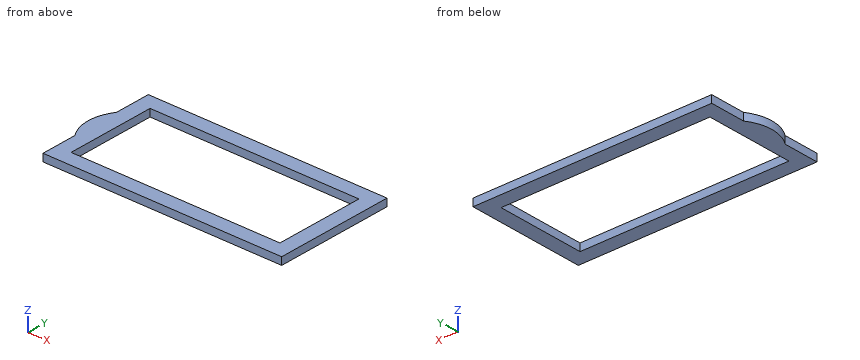
from build123d import *

# Parameters (mm, degrees)
F1_DEPTH = 1.5875


with BuildPart() as f1:
    # F0 (on Top) → F1 (new body)
    with BuildSketch(Plane.XY):
        with BuildLine():
            Line((0, 7.6798842145), (0, 0))
            Line((0, 0), (50.8, 0))
            Line((50.8, 0), (50.8, 25.4))
            Line((50.8, 25.4), (0, 25.4))
            Line((0, 25.4), (0, 17.7201157855))
            ThreePointArc((0, 17.7201157855), (1.4190494999, 19.2926118305), (3.175, 20.4771299333))
            Line((3.175, 20.4771299333), (3.175, 22.225))
            Line((3.175, 22.225), (47.625, 22.225))
            Line((47.625, 22.225), (47.625, 3.175))
            Line((47.625, 3.175), (3.175, 3.175))
            Line((3.175, 3.175), (3.175, 4.9228700667))
            ThreePointArc((3.175, 4.9228700667), (1.4190494999, 6.1073881695), (0, 7.6798842145))
        make_face()
        with BuildLine():
            ThreePointArc((0, 17.7201157855), (-1.5875, 12.7), (0, 7.6798842145))
            Line((0, 7.6798842145), (0, 17.7201157855))
        make_face()
        with BuildLine():
            Line((0, 17.7201157855), (0, 7.6798842145))
            ThreePointArc((0, 7.6798842145), (1.4190494999, 6.1073881695), (3.175, 4.9228700667))
            Line((3.175, 4.9228700667), (3.175, 20.4771299333))
            ThreePointArc((3.175, 20.4771299333), (1.4190494999, 19.2926118305), (0, 17.7201157855))
        make_face()
    extrude(amount=F1_DEPTH)


solid = f1.part
Input: part model. Units: mm. Frame: model coordinates. Round coordinates to 2 decimals unless told otherwise and drop trailing zeros. Order: outer loops, then holes, each group sorted by start corner. A loop starts at its lowest first (then second) coordinate and runs counter-clockwise, first axis right, second up. Notation, with made-up numbers: (5.25, -9.5) - (14.25, -9.5) arc R20 ccw to (14.25, -5.5) - close; hole circle Ø8 at (76, -40). An arc over 180 degrees is marked (long way). Use a Markdown table: item, result.
1. Section D-D on y = 2.5. Return the cut outline in (x, z), then the cut area to 3 significant figures.
Evaluation:
| item | result |
|---|---|
| outline | (0, 0) - (50.8, 0) - (50.8, 1.59) - (0, 1.59) - close |
| area | 80.6 mm^2 |
2. Section C-C on y = 18.25. Return the cut outline in (x, z) (1 decimal).
Evaluation:
| item | result |
|---|---|
| outline | (0, 0) - (3.2, 0) - (3.2, 1.6) - (0, 1.6) - close; (47.6, 0) - (50.8, 0) - (50.8, 1.6) - (47.6, 1.6) - close |
3. Material intervals for probe 1 along Y at (x, z) = (17, 0.1) (3 decimals); probe 2 along X at (y, z) = (7, 1.5) (3 decimals); probe 3 along X at (y, z) = (16, 1.2) (3 decimals), sorted ascending.
Evaluation:
| item | result |
|---|---|
| probe 1 | 0 to 3.175, 22.225 to 25.4 |
| probe 2 | 0 to 3.175, 47.625 to 50.8 |
| probe 3 | -0.94 to 3.175, 47.625 to 50.8 |
4. Section B-B on x = 10. Return the cut outline in (y, z) (1 decimal).
Evaluation:
| item | result |
|---|---|
| outline | (0, 0) - (3.2, 0) - (3.2, 1.6) - (0, 1.6) - close; (22.2, 0) - (25.4, 0) - (25.4, 1.6) - (22.2, 1.6) - close |
5. Section A-A on z = 0.8. Return the cut outline in (x, y) (1 decimal), then the cut area to 3 significant figures.
Evaluation:
| item | result |
|---|---|
| outline | (0, 0) - (50.8, 0) - (50.8, 25.4) - (0, 25.4) - (0, 17.7) arc R8.7 ccw to (0, 7.7) - close; hole (3.2, 3.2) - (47.6, 3.2) - (47.6, 22.2) - (3.2, 22.2) - close |
| area | 454 mm^2 |
